Source: CAD feature listing. Evaluate the final solid. Frame: model axes, mm. A direction names the side the tool comes from. Round coordinates to 2 decimals unless told otherwise and drop trailing zeros. Write each loop counter-clockwise with the first axis right and the second up, starting at its lowest first coordinate (ties: lowest second). Pieces come first, ordered by that corner, then holes.
from build123d import *

# Parameters (mm, degrees)
EXTRUDE_1_DEPTH     = 4
CUT_EXTRUDE_START   = 4
SKETCH_2_R          = 2.2
CUT_EXTRUDE_2_DEPTH = 2
SKETCH_3_R          = 2.2
CUT_EXTRUDE_3_DEPTH = 2
SKETCH_4_R          = 1.2
CUT_EXTRUDE_4_DEPTH = 22.260291625
SKETCH_5_R          = 1.2
CUT_EXTRUDE_5_DEPTH = 22.260291625
FILLET_1_R          = 1
SKETCH_6_W          = 26
SKETCH_6_H          = 6
CUT_EXTRUDE_8_DEPTH = 0.4


with BuildPart() as part:
    # 草圖1 → 填料-伸長1 (new body)
    with BuildSketch(Plane(origin=(0, 0, 0), x_dir=(1, 0, 0), z_dir=(0, 1, 0))):
        Polygon((-13, -6), (20, -6), (20, 6), (-7, 6), (-7, 0), (-13, 0), align=None)
    extrude(amount=EXTRUDE_1_DEPTH)

    # 草圖2 → 除料-伸長2 (cut)
    with BuildSketch(Plane(origin=(0, 0, 0), x_dir=(1, 0, 0), z_dir=(0, 1, 0)).offset(CUT_EXTRUDE_START)):
        with Locations(Location((-4, 3.015018989, 0), (0, 0, 270))):
            Circle(SKETCH_2_R)
    extrude(amount=-CUT_EXTRUDE_2_DEPTH, mode=Mode.SUBTRACT)

    # 草圖3 → 除料-伸長3 (cut)
    with BuildSketch(Plane(origin=(0, 0, 0), x_dir=(1, 0, 0), z_dir=(0, 1, 0)).offset(CUT_EXTRUDE_START)):
        with Locations(Location((16, -3, 0), (0, 0, 270))):
            Circle(SKETCH_3_R)
        with Locations(Location((16, 3, 0), (0, 0, 90))):
            Circle(SKETCH_3_R)
    extrude(amount=-CUT_EXTRUDE_3_DEPTH, mode=Mode.SUBTRACT)

    # 草圖4 → 除料-伸長4 (cut, through all)
    with BuildSketch(Plane(origin=(0, 0, 0), x_dir=(1, 0, 0), z_dir=(0, 1, 0))):
        with Locations(Location((-4, 3.015018989, 0), (0, 0, 270))):
            Circle(SKETCH_4_R)
        with Locations(Location((16, -3, 0), (0, 0, 270))):
            Circle(SKETCH_4_R)
    extrude(amount=CUT_EXTRUDE_4_DEPTH, mode=Mode.SUBTRACT)

    # 草圖5 → 除料-伸長5 (cut, through all)
    with BuildSketch(Plane(origin=(0, 0, 0), x_dir=(1, 0, 0), z_dir=(0, 1, 0))):
        with Locations(Location((16, 3, 0), (0, 0, 90))):
            Circle(SKETCH_5_R)
    extrude(amount=CUT_EXTRUDE_5_DEPTH, mode=Mode.SUBTRACT)

    # 圓角1
    # the kernel refuses this fillet: 1 mm, written as the material it takes off along each edge
    with BuildSketch(Plane(origin=(19, 3, 5), x_dir=(1, 0, 0), z_dir=(0, 0, 1))) as fillet_1_piece_1_section:
        Polygon((0, 0), (FILLET_1_R, 0), (FILLET_1_R, FILLET_1_R), (0, FILLET_1_R), align=None)
    fillet_1_piece_1 = extrude(amount=FILLET_1_R, mode=Mode.PRIVATE)
    fillet_1_piece_1 = fillet_1_piece_1 - Plane(origin=(19, 3, 5), x_dir=(-0.7071067811865475, -0.7071067811865475, 0), z_dir=(0, 0, 1)) * Sphere(FILLET_1_R, mode=Mode.PRIVATE)
    add(fillet_1_piece_1, mode=Mode.SUBTRACT)
    with BuildSketch(Plane(origin=(19, 3, -5), x_dir=(0, 1, 0), z_dir=(1, 0, 0))) as fillet_1_piece_2_section:
        Polygon((0, 0), (FILLET_1_R, 0), (FILLET_1_R, -FILLET_1_R), (0, -FILLET_1_R), align=None)
    fillet_1_piece_2 = extrude(amount=FILLET_1_R, mode=Mode.PRIVATE)
    fillet_1_piece_2 = fillet_1_piece_2 - Plane(origin=(19, 3, -5), x_dir=(0, -0.7071067811865475, 0.7071067811865475), z_dir=(1, 0, 0)) * Sphere(FILLET_1_R, mode=Mode.PRIVATE)
    add(fillet_1_piece_2, mode=Mode.SUBTRACT)
    with BuildSketch(Plane(origin=(-12, 3, 1), x_dir=(0, 1, 0), z_dir=(-1, 0, 0))) as fillet_1_piece_3_section:
        Polygon((0, 0), (FILLET_1_R, 0), (FILLET_1_R, FILLET_1_R), (0, FILLET_1_R), align=None)
    fillet_1_piece_3 = extrude(amount=FILLET_1_R, mode=Mode.PRIVATE)
    fillet_1_piece_3 = fillet_1_piece_3 - Plane(origin=(-12, 3, 1), x_dir=(0, -0.7071067811865475, 0.7071067811865475), z_dir=(-1, 0, 0)) * Sphere(FILLET_1_R, mode=Mode.PRIVATE)
    add(fillet_1_piece_3, mode=Mode.SUBTRACT)
    with BuildSketch(Plane(origin=(-6, 3, -5), x_dir=(0, 0, -1), z_dir=(0, 1, 0))) as fillet_1_piece_4_section:
        Polygon((0, 0), (FILLET_1_R, 0), (FILLET_1_R, FILLET_1_R), (0, FILLET_1_R), align=None)
    fillet_1_piece_4 = extrude(amount=FILLET_1_R, mode=Mode.PRIVATE)
    fillet_1_piece_4 = fillet_1_piece_4 - Plane(origin=(-6, 3, -5), x_dir=(0.7071067811865475, 0, 0.7071067811865477), z_dir=(0, 1, 0)) * Sphere(FILLET_1_R, mode=Mode.PRIVATE)
    add(fillet_1_piece_4, mode=Mode.SUBTRACT)
    with BuildSketch(Plane(origin=(-12, 3, 5), x_dir=(-1, 0, 0), z_dir=(0, 0, 1))) as fillet_1_piece_5_section:
        Polygon((0, 0), (FILLET_1_R, 0), (FILLET_1_R, -FILLET_1_R), (0, -FILLET_1_R), align=None)
    fillet_1_piece_5 = extrude(amount=FILLET_1_R, mode=Mode.PRIVATE)
    fillet_1_piece_5 = fillet_1_piece_5 - Plane(origin=(-12, 3, 5), x_dir=(0.7071067811865475, -0.7071067811865475, 0), z_dir=(0, 0, 1)) * Sphere(FILLET_1_R, mode=Mode.PRIVATE)
    add(fillet_1_piece_5, mode=Mode.SUBTRACT)
    with BuildSketch(Plane(origin=(20, 4, 5), x_dir=(0, -1, 0), z_dir=(0, 0, -1))) as fillet_1_piece_6:
        with BuildLine():
            CenterArc((FILLET_1_R, FILLET_1_R), FILLET_1_R, 180, 90)
            Line((0, FILLET_1_R), (0, 0))
            Line((0, 0), (FILLET_1_R, 0))
        make_face()
    extrude(amount=10, mode=Mode.SUBTRACT)
    with BuildSketch(Plane(origin=(-13, -2.5, 0), x_dir=(0, 0, 1), z_dir=(0, 1, 0)), Plane(origin=(-13, -2.5, 6), x_dir=(1, 0, 0), z_dir=(0, 1, 0))) as fillet_1_piece_7:
        with BuildLine():
            CenterArc((FILLET_1_R, FILLET_1_R), FILLET_1_R, 180, 90)
            Line((0, FILLET_1_R), (0, 0))
            Line((0, 0), (FILLET_1_R, 0))
        make_face()
    extrude(amount=5.5, mode=Mode.SUBTRACT)
    with BuildSketch(Plane(origin=(-7, -2.5, -6), x_dir=(1, 0, 0), z_dir=(0, 1, 0)), Plane(origin=(20, -2.5, -6), x_dir=(0, 0, 1), z_dir=(0, 1, 0)), Plane(origin=(20, -2.5, 6), x_dir=(-1, 0, 0), z_dir=(0, 1, 0))) as fillet_1_piece_8:
        with BuildLine():
            CenterArc((FILLET_1_R, -FILLET_1_R), FILLET_1_R, 90, 90)
            Line((0, -FILLET_1_R), (0, 0))
            Line((0, 0), (FILLET_1_R, 0))
        make_face()
    extrude(amount=5.5, mode=Mode.SUBTRACT)
    with BuildSketch(Plane(origin=(19, 4, -6), x_dir=(0, 0, 1), z_dir=(-1, 0, 0))) as fillet_1_piece_9:
        with BuildLine():
            CenterArc((FILLET_1_R, -FILLET_1_R), FILLET_1_R, 90, 90)
            Line((0, -FILLET_1_R), (0, 0))
            Line((0, 0), (FILLET_1_R, 0))
        make_face()
    extrude(amount=25, mode=Mode.SUBTRACT)
    with BuildSketch(Plane(origin=(-7, 4, -5), x_dir=(1, 0, 0), z_dir=(0, 0, 1)), Plane(origin=(-7, 4, 0), x_dir=(0, 0, 1), z_dir=(-1, 0, 0))) as fillet_1_piece_10:
        with BuildLine():
            CenterArc((FILLET_1_R, -FILLET_1_R), FILLET_1_R, 90, 90)
            Line((0, -FILLET_1_R), (0, 0))
            Line((0, 0), (FILLET_1_R, 0))
        make_face()
    extrude(amount=5, mode=Mode.SUBTRACT)
    with BuildSketch(Plane(origin=(-13, 4, 1), x_dir=(0, -1, 0), z_dir=(0, 0, 1))) as fillet_1_piece_11:
        with BuildLine():
            CenterArc((FILLET_1_R, FILLET_1_R), FILLET_1_R, 180, 90)
            Line((0, FILLET_1_R), (0, 0))
            Line((0, 0), (FILLET_1_R, 0))
        make_face()
    extrude(amount=4, mode=Mode.SUBTRACT)
    with BuildSketch(Plane(origin=(-12, 4, 6), x_dir=(0, -1, 0), z_dir=(1, 0, 0))) as fillet_1_piece_12:
        with BuildLine():
            CenterArc((FILLET_1_R, FILLET_1_R), FILLET_1_R, 180, 90)
            Line((0, FILLET_1_R), (0, 0))
            Line((0, 0), (FILLET_1_R, 0))
        make_face()
    extrude(amount=31, mode=Mode.SUBTRACT)
    with BuildSketch(Plane(origin=(-4.5, 4, 0), x_dir=(0, 0, 1), z_dir=(-1, 0, 0))) as fillet_1_piece_13a_section:
        with BuildLine():
            CenterArc((FILLET_1_R, -FILLET_1_R), FILLET_1_R, 90, 90)
            Line((0, -FILLET_1_R), (0, 0))
            Line((0, 0), (FILLET_1_R, 0))
        make_face()
    fillet_1_piece_13a = extrude(amount=7.5, mode=Mode.PRIVATE)
    fillet_1_piece_13a = split(fillet_1_piece_13a, bisect_by=Plane(origin=(-7, 3.773604886, 0.226395114), z_dir=(1, 0, 0)), keep=Keep.TOP, mode=Mode.PRIVATE)
    with BuildSketch(Plane(origin=(-7, 4, -5), x_dir=(1, 0, 0), z_dir=(0, 0, 1))) as fillet_1_piece_13b_section:
        with BuildLine():
            CenterArc((FILLET_1_R, -FILLET_1_R), FILLET_1_R, 90, 90)
            Line((0, -FILLET_1_R), (0, 0))
            Line((0, 0), (FILLET_1_R, 0))
        make_face()
    fillet_1_piece_13b = extrude(amount=7.5, mode=Mode.PRIVATE)
    fillet_1_piece_13b = split(fillet_1_piece_13b, bisect_by=Plane(origin=(-6.773604886, 3.773604886, 0), z_dir=(0, 0, 1)), keep=Keep.TOP, mode=Mode.PRIVATE)
    fillet_1_piece_13 = fillet_1_piece_13a & fillet_1_piece_13b
    add(fillet_1_piece_13, mode=Mode.SUBTRACT)

    # 草圖6 → 除料-伸長8 (cut)
    with BuildSketch(Plane(origin=(0, 0, 0), x_dir=(1, 0, 0), z_dir=(0, 1, 0))):
        with Locations((0, -3)):
            Rectangle(SKETCH_6_W, SKETCH_6_H)
    extrude(amount=CUT_EXTRUDE_8_DEPTH, mode=Mode.SUBTRACT)


solid = part.part
1) Section query A-A on y = 1.25. Return the cut outline in (x, z), then the cut area to 3 significant figures.
Taken from the geometry:
outline: (-13, 1) arc R1 ccw to (-12, 0) - (-7, 0) - (-7, -5) arc R1 ccw to (-6, -6) - (19, -6) arc R1 ccw to (20, -5) - (20, 5) arc R1 ccw to (19, 6) - (-12, 6) arc R1 ccw to (-13, 5) - close; hole circle Ø2.4 at (-4, -3.02); hole circle Ø2.4 at (16, -3); hole circle Ø2.4 at (16, 3)
area: 345 mm2
2) Section query B-B on x = 16. Return the cut outline in (y, z), then the cut area to 3 significant figures.
Taken from the geometry:
outline: (0, -6) - (3, -6) arc R1 ccw to (3.98, -5.2) - (2, -5.2) - (2, -4.2) - (0, -4.2) - close; (0, -1.8) - (2, -1.8) - (2, -0.8) - (4, -0.8) - (4, 0.8) - (2, 0.8) - (2, 1.8) - (0, 1.8) - close; (0, 4.2) - (2, 4.2) - (2, 5.2) - (3.98, 5.2) arc R1 ccw to (3, 6) - (0, 6) - close
area: 20.4 mm2
3) Material intervals for line 1 (X direction, y = 3, z = -3); line 2 (Z direction, x = 16, y = 2.95); line 3 (Z direction, x = 16, y = 1.15), sorted ascending.
Taken from the geometry:
line 1: x = -7 to -6.2, -1.8 to 13.8, 18.2 to 20
line 2: z = -6 to -5.2, -0.8 to 0.8, 5.2 to 6
line 3: z = -6 to -4.2, -1.8 to 1.8, 4.2 to 6
4) Section query D-D on x = 5. Return the cut outline in (y, z).
Taken from the geometry:
outline: (0, -6) - (3, -6) arc R1 ccw to (4, -5) - (4, 5) arc R1 ccw to (3, 6) - (0.4, 6) - (0.4, 0) - (0, 0) - close
5) Reachability of faces 1 (the face through (-6.699, 3.715, -2.042)), 2 (the face through (15, 2, 4)), 3 (the face through (19.699, 3.715, 0.07)), 4 (the face through (-9, 2, 0)) from +Z, -Z, +X, -X, +Y, -Y: full face, straight path, thin tool, end or side. Return the list, or none.
Taken from the geometry:
face 1: -Z, -X, +Y
face 2: +Y
face 3: +Z, -Z, +X, +Y
face 4: -Z, -X, +Y, -Y
6) Pull-direction query (X, two-part tool) for faces 5 (the face through (19.715, 1.479, -5.699)), 6 (the face through (0, 0.4, 3)), 7 (the face through (18.148, 3.014, -2.523)); classes: released by +X, released by -X, zero draft, split by the parting line, or undercut.
Taken from the geometry:
face 5: released by +X
face 6: zero draft
face 7: undercut
7) Contact query for flat-ended pins moving along their axis: P1, Ø3, axis at x = 16, z = -3, coming from the +Y side; P2, Ø1, axis at x = 1.5, z = 4, coming from the -Y side; P3, Ø1.4, axis at x = -4, z = -3.02, coming from the +Y side; P4, Ø1.5, axis at y = 1.5, z = -3.5, coming from the -X side. Output: stop coordinate, or through.
Taken from the geometry:
P1: stops at y = 2
P2: stops at y = 0.4
P3: passes through
P4: stops at x = -7
8) Section query C-C on z = -3. Return the cut outline in (x, y).
Taken from the geometry:
outline: (-7, 0) - (-5.2, 0) - (-5.2, 2) - (-6.2, 2) - (-6.2, 3.98) arc R1 ccw to (-7, 3) - close; (-2.8, 0) - (14.8, 0) - (14.8, 2) - (13.8, 2) - (13.8, 4) - (-1.8, 4) - (-1.8, 2) - (-2.8, 2) - close; (17.2, 0) - (20, 0) - (20, 3) arc R1 ccw to (19, 4) - (18.2, 4) - (18.2, 2) - (17.2, 2) - close
